from build123d import *

# Parameters (mm, degrees)
F0_R     = 3.175
F0_W     = 5.842
F0_H     = 12.7
F2_DEPTH = 6.35
F3_DEPTH = 7.62


with BuildPart() as f1:
    # F0 (on Front) → F1 (revolve)
    with BuildSketch(Plane.XZ):
        Polygon((5.842, 12.7), (5.842, 0), (66.294, 0), (66.294, 12.7), (56.134, 12.7), (56.134, 10.16), (10.16, 10.16), (10.16, 12.7), align=None)
    revolve(axis=Axis((33.147, 0, 0), (-1, 0, 0)))

    # F0 (on Front) → F2 (join)
    with BuildSketch(Plane.XZ):
        with BuildLine():
            ThreePointArc((-8.1826630726, -5.5069827884), (-3.1957909266, -4.5493385486), (-0.9398, 0))
            ThreePointArc((-0.9398, 0), (-4.5919612295, 5.3297205562), (-10.8806298187, 3.8475430269))
            ThreePointArc((-10.8806298187, 3.8475430269), (-12.1459778134, -1.5837270034), (-8.1826630726, -5.5069827884))
        make_face()
        with Locations((-6.6548, 0)):
            Circle(F0_R, mode=Mode.SUBTRACT)
        with BuildLine():
            Line((5.842, 0), (0, 0))
            Line((0, 0), (-0.9398, 0))
            ThreePointArc((-0.9398, 0), (-3.1957909266, -4.5493385486), (-8.1826630726, -5.5069827884))
            Line((-8.1826630726, -5.5069827884), (5.842, -9.398))
            Line((5.842, -9.398), (5.842, 0))
        make_face()
        with BuildLine():
            Line((-0.9398, 0), (0, 0))
            Line((0, 0), (0, 12.7))
            Line((0, 12.7), (5.842, 12.7))
            Line((5.842, 12.7), (5.842, 15.24))
            Line((5.842, 15.24), (-0.508, 15.24))
            Line((-0.508, 15.24), (-10.8806298187, 3.8475430269))
            ThreePointArc((-10.8806298187, 3.8475430269), (-4.5919612295, 5.3297205562), (-0.9398, 0))
        make_face()
        with Locations((2.921, 6.35)):
            Rectangle(F0_W, F0_H)
    extrude(amount=F2_DEPTH)

    # F3 (add): a face of the model
    f3_faces = [f1.faces().sort_by_distance(p)[0] for p in [
        (10.16, 0, -10.5192102448),
    ]]
    extrude(f3_faces, amount=F3_DEPTH)


solid = f1.part
The listing builds one solid part. Answer for the finished solid, in the listing's coordinates (mm). A direction names the side the tool comes from. Round coordinates to 2 decimals unless told otherwise and drop trailing zeros. Order: outer loops, then holes, each group sorted by start corner. A loop starts at its lowest first (then second) coordinate and runs counter-clockwise, first axis right, second up. Notation, with made-up numbers: M 72.5,79.25 L 104.5,79.25 A17 cw 104.5,89.25 Z; hole C 38,32 d11. An arc over 180 degrees is marked long. Answer in a Markdown table with one row per item. Add a question column.
1) The part is cut by section C-C on x = 60. Determine the outline of the cut face in (y, z), plus the area to 3 significant figures.
2) Consider line 1 along X through (y, z) = (10.25, -0.25); line 2 along X through (y, z) = (4.25, 0); line 3 along Z through (x, y) = (1.5, -5). Determine where each line is inside the solid, lowest interval first. Write a range as from..to.
3) Which of the six approach directions +Z, -Z, +X, -X, +Y, -Y give full straight-line access (tool end or side, diameter ignored) to faces 1 (the face through (3, -3, 15.24)), 2 (the face through (17.78, 9, 6)), 3 (the face through (-1, 0, 3))?
4) Determine the mould class of faces 4 (the face through (-1, -6.35, 3)), 5 (the face through (5.842, -3, 14)), 6 (the face through (-5.622, -3.131, 9.624)), 7 (the face through (56.134, 9, -6)) for opening direction X: pulls with the +X half, pulls with the -X half, needs draft (parallel to the pull), parting line crosses it, or undercut.
5) Flat-ended cylindrical pins translate along their axes: pin 1 Ø1.5 at (x, z) = (51, -4) entering from +Y; pin 2 Ø3 at (y, z) = (-7, -5.5) entering from -X; pin 3 Ø1.5 at (x, z) = (-1, 3.5) entering from +Y; pin 4 Ø4 at (x, z) = (-6.65, 0) entering from -Y. Find the tip coordinate at first contact, or state that the pin passes through.
6) The part is cut by section D-D on y = -8.5. Determine the outline of the cut face in (x, z).
7) The part is cut by section A-A on z = 0. Determine the outline of the cut face in (x, y), plus the area to 3 significant figures.
8) The part is cut by section B-B on y = -3. Determine the outline of the cut face in (x, z) (3 decimals), plus the area to 3 significant figures.
Findings below:
| question | item | result |
|---|---|---|
| 1 | outline | C 0,0 d25.4 |
| 1 | area | 507 mm² |
| 2 | line 1 | x = 5.84..17.78, 56.13..66.29 |
| 2 | line 2 | x = 5.84..66.29 |
| 2 | line 3 | z = -8.19..15.24 |
| 3 | face 1 | +Z, +X, -X, +Y, -Y |
| 3 | face 2 | none |
| 3 | face 3 | +Z, -Z, -X, +Y |
| 4 | face 4 | needs draft |
| 4 | face 5 | pulls with the +X half |
| 4 | face 6 | pulls with the -X half |
| 4 | face 7 | undercut |
| 5 | pin 1 | stops at y = 9.63 |
| 5 | pin 2 | stops at x = -10.59 |
| 5 | pin 3 | stops at y = 0 |
| 5 | pin 4 | passes through |
| 6 | outline | M 5.84,-9.44 L 17.78,-9.44 L 17.78,-5.57 L 56.13,-5.57 L 56.13,-9.44 L 66.29,-9.44 L 66.29,9.44 L 56.13,9.44 L 56.13,5.57 L 17.78,5.57 L 17.78,9.44 L 5.84,9.44 Z |
| 7 | outline | M -12.37,-6.35 L -9.83,-6.35 L -9.83,0 L -12.37,0 Z; M -3.48,-6.35 L 5.84,-6.35 L 5.84,-12.7 L 17.78,-12.7 L 17.78,-10.16 L 56.13,-10.16 L 56.13,-12.7 L 66.29,-12.7 L 66.29,12.7 L 56.13,12.7 L 56.13,10.16 L 17.78,10.16 L 17.78,12.7 L 5.84,12.7 L 5.84,0 L -3.48,0 Z |
| 7 | area | 1,420 mm² |
| 8 | outline | M -10.881,3.848 A5.715 ccw -8.183,-5.507 L 5.842,-9.398 L 5.842,-12.341 L 17.78,-12.341 L 17.78,-9.707 L 56.134,-9.707 L 56.134,-12.341 L 66.294,-12.341 L 66.294,12.341 L 56.134,12.341 L 56.134,9.707 L 17.78,9.707 L 17.78,12.341 L 5.842,12.341 L 5.842,15.24 L -0.508,15.24 Z; hole C -6.655,0 d6.35 |
| 8 | area | 1,580 mm² |
